Here's how the part is built. I have some questions about the finished solid (model axes, mm). Coordinates: 2 decimals unless noted, no trailing zeros. Loops run counter-clockwise (first coordinate to the right, second up) from the corner with the lowest first, then second, coordinate; pieces in that order, holes last. Notation, with made-up numbers: (-38.5, -2) -> (-16.5, -2) arc R9 cw to (-16.5, 9) -> close; hole circle Ø4 at (80, 12). An arc over 180 degrees is marked (long way). Answer as a JSON object with one key per item and string values. Group by question number.
1) I want a section at B-B (z = -87). Write out the boundary of the cut face in (x, y).
2) I want a section at C-C (x = 75). Write out the boundary of the cut face in (y, z).
3) I want a section at A-A (y = 3.25). Write out the boundary of the cut face in (x, z).
4) I need wall thicknesses on probe 1 along X at (y, z) = (3.5, -88); probe 2 along X at (y, z) = (1.5, -94.5); probe 3 along Z at (x, y) = (77, 4). Which ranges of each line are inside material? Lowest first, please. Write a range as [from, to].
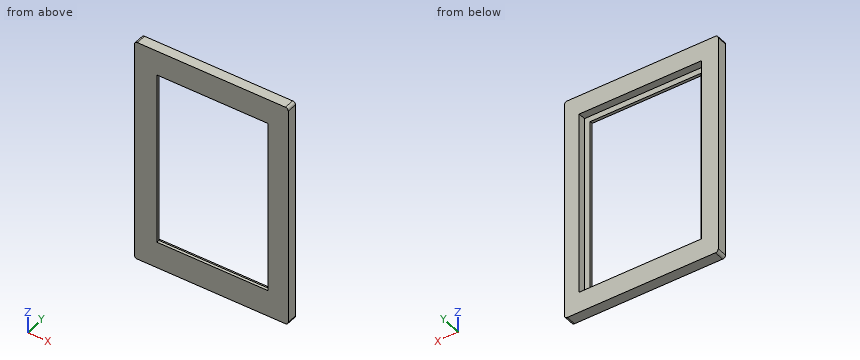
Autodesk Inventor part; units mm, degrees
ref_plane "YZ Plane" through (0, 0, 0) normal (1, 0, 0) x (0, 1, 0)
ref_plane "XZ Plane" through (0, 0, 0) normal (0, 1, 0) x (-1, 0, 0)
ref_plane "XY Plane" through (0, 0, 0) normal (0, 0, 1) x (1, 0, 0)
sketch "草图1" plane through (0, 0, 0) normal (0, 1, 0) x (-1, 0, 0)
  line L0 (0, 0) -> (0, -158)
  line L1 (0, -158) -> (-108, -158)
  line L2 (-108, -158) -> (-108, 0)
  line L3 (-108, 0) -> (0, 0)
  line L4 (-54.65, -78.4) -> (-11.65, -78.4)
  line L5 (-11.65, -78.4) -> (-11.65, -143.4)
  line L6 (-11.65, -143.4) -> (-97.65, -143.4)
  line L7 (-97.65, -143.4) -> (-97.65, -13.4)
  line L8 (-97.65, -13.4) -> (-11.65, -13.4)
  line L9 (-11.65, -13.4) -> (-11.65, -78.4)
  dimension "d0" = 158
  dimension "d1" = 108
  dimension "d2" = 43
  dimension "d4" = 65
  dimension "d5" = 86
  dimension "d6" = 130
extrude "拉伸1" add sketch "草图1" along normal blind 7.2
fillet "圆角1" radius 2 4 edges at (108, 3.6, 0) (108, 3.6, -158) (0, 3.6, 0) (0, 3.6, -158)
sketch "草图2" plane through (0, 0, 0) normal (0, -1, 0) x (1, 0, 0)
  line L0 (11.65, -143.4) -> (97.65, -143.4)
  line L1 (11.65, -143.4) -> (11.65, -139.4)
  line L2 (11.65, -13.4) -> (11.65, -143.4)
  line L3 (11.65, -139.4) -> (15.65, -139.4)
  line L4 (15.65, -139.4) -> (93.65, -139.4)
  line L5 (93.65, -139.4) -> (93.65, -17.4)
  line L6 (93.65, -17.4) -> (15.65, -17.4)
  line L7 (15.65, -17.4) -> (15.65, -139.4)
  line L8 (97.65, -13.4) -> (11.65, -13.4)
  line L9 (11.65, -143.4) -> (97.65, -143.4)
  line L10 (97.65, -143.4) -> (97.65, -13.4)
  line L11 (97.65, -13.4) -> (11.65, -13.4)
  line L12 (11.65, -13.4) -> (11.65, -143.4)
  point P0 (0, 0)
  point P1 (97.65, -143.4)
  dimension "d10" = 4
  dimension "d11" = 4
  dimension "d12" = 78
  dimension "d13" = 122
extrude "拉伸2" add sketch "草图2" against normal blind 2
equation "\"折弯半径\" = 厚度"
equation "\"折弯释压宽度\" = 厚度"
equation "\"折弯释压深度\" = 0.5 * 厚度"
equation "\"拐角释压尺寸\" = 4 * 厚度"
equation "\"最小余量\" = 2 * 厚度"
equation "\"过渡半径\" = 折弯半径"
equation "\"Jacobi半径尺寸\" = 折弯半径"
equation "\"间隙大小\" = 厚度"
properties part number "plate-holder"
Determined:
{
 "1": {"outline": "(0, 0) -> (15.65, 0) -> (15.65, 2) -> (11.65, 2) -> (11.65, 7.2) -> (0, 7.2) -> close; (93.65, 0) -> (108, 0) -> (108, 7.2) -> (97.65, 7.2) -> (97.65, 2) -> (93.65, 2) -> close"},
 "2": {"outline": "(0, -158) -> (7.2, -158) -> (7.2, -143.4) -> (2, -143.4) -> (2, -139.4) -> (0, -139.4) -> close; (0, -17.4) -> (2, -17.4) -> (2, -13.4) -> (7.2, -13.4) -> (7.2, 0) -> (0, 0) -> close"},
 "3": {"outline": "(0, -156) arc R2 ccw to (2, -158) -> (106, -158) arc R2 ccw to (108, -156) -> (108, -2) arc R2 ccw to (106, 0) -> (2, 0) arc R2 ccw to (0, -2) -> close; hole (11.65, -143.4) -> (97.65, -143.4) -> (97.65, -13.4) -> (11.65, -13.4) -> close"},
 "4": {"probe 1": "[0, 11.65], [97.65, 108]", "probe 2": "[0, 15.65], [93.65, 108]", "probe 3": "[-158, -143.4], [-13.4, 0]"}
}
